For this review, use the dimensioned drawing (mm, ordinates from the lowest corner) and the shaded views. Give positions to 0.01 mm unless a question says otherwise; leave off trailing zeros. Order: outer loops, then holes, each group sorted by start corner. A loop starts at its lowest first (then second) coordinate and runs counter-clockwise, first axis right, second up. Notation, with made-up numbers: (31, -2.5) - (90, -2.5) arc R23 ccw to (90, 29.5) - close; hole circle Ø9 at (-25, 87). An arc over 180 degrees is marked (long way). Answer as CSV lines item,"result". Start each with the question number.
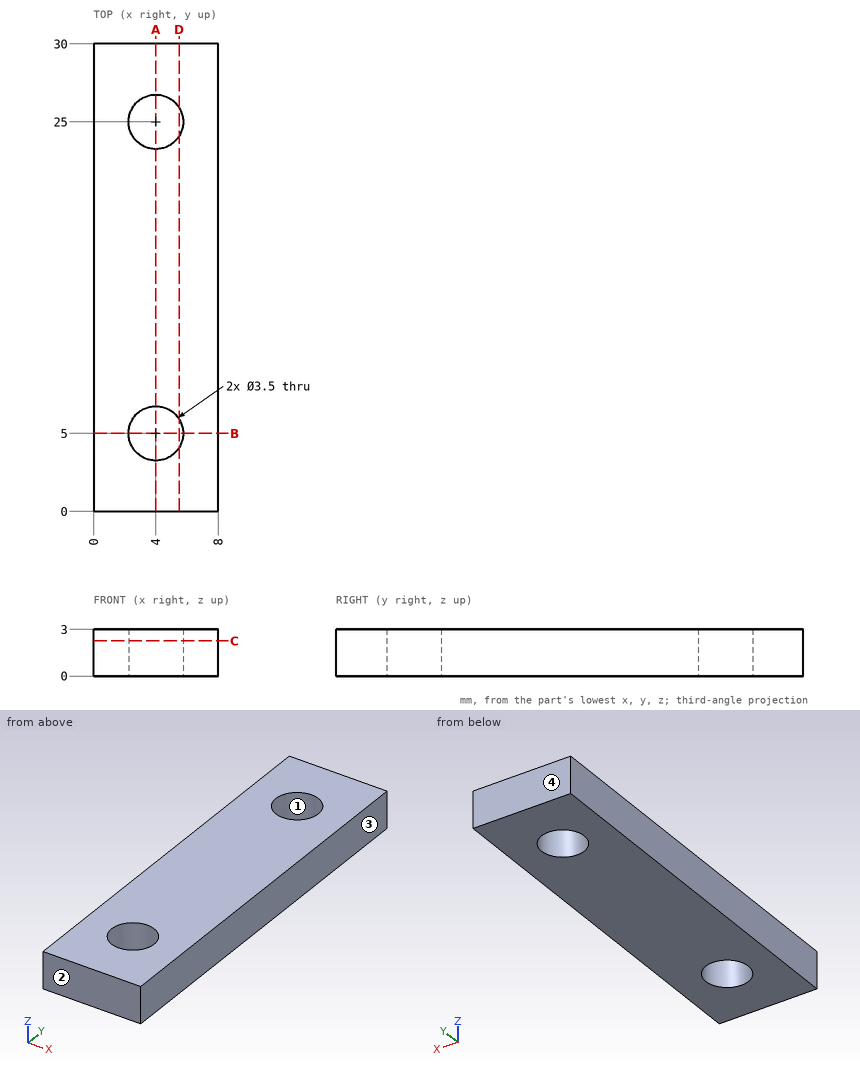
Item 1: For line 1 along X through (y, z) = (5, 1.9); line 2 along Y through (x, z) = (4, 1.7); line 3 along Y through (x, z) = (2.75, 1.1), list the stretches that pass through material, from the lowest coordinate up.
Item 2: Take a section at B-B on y = 5. Write out the cut boundary in (x, z).
Item 3: Take a section at C-C on z = 2.25. Write out the cut boundary in (x, y), and give its area (3 significant figures).
Item 4: Take a section at D-D on x = 5.5. Write out the cut boundary in (y, z).
Item 5: Take a section at A-A on x = 4. Write out the cut boundary in (y, z).
Item 6: Mouldability with a two-part tool opening along Y and no side actions: class the marked faces 1, 2, 3 and 4 as released by +Y, released by -Y, zero draft, split by the parting line, or undercut.
Data:
1,line 1,"x = 0 to 2.25, 5.75 to 8"
1,line 2,"y = 0 to 3.25, 6.75 to 23.25, 26.75 to 30"
1,line 3,"y = 0 to 3.78, 6.22 to 23.78, 26.22 to 30"
2,outline,"(0, 0) - (2.25, 0) - (2.25, 3) - (0, 3) - close; (5.75, 0) - (8, 0) - (8, 3) - (5.75, 3) - close"
3,outline,"(0, 0) - (8, 0) - (8, 30) - (0, 30) - close; hole circle Ø3.5 at (4, 5); hole circle Ø3.5 at (4, 25)"
3,area,"221 mm^2"
4,outline,"(0, 0) - (4.1, 0) - (4.1, 3) - (0, 3) - close; (5.9, 0) - (24.1, 0) - (24.1, 3) - (5.9, 3) - close; (25.9, 0) - (30, 0) - (30, 3) - (25.9, 3) - close"
5,outline,"(0, 0) - (3.25, 0) - (3.25, 3) - (0, 3) - close; (6.75, 0) - (23.25, 0) - (23.25, 3) - (6.75, 3) - close; (26.75, 0) - (30, 0) - (30, 3) - (26.75, 3) - close"
6,face 1,"undercut"
6,face 2,"released by -Y"
6,face 3,"zero draft"
6,face 4,"released by +Y"
